Print and shaded views of the part. All mm, measured from the part's lowest x, y and z. A direction names the side the tool comes from. Round coordinates to 2 decimals unless told otherwise and drop trailing zeros. Write each loop counter-clockwise with the first axis right and the second up, starting at its lowest first coordinate (ties: lowest second). Pieces come first, ordered by that corner, then holes. Notation, with made-up numbers: (88, 10.25) - (139, 10.25) arc R31 cw to (139, 41.25) - close; hole circle Ø6 at (25.25, 6.5). An arc over 180 degrees is marked (long way). One line per item, written item: value.
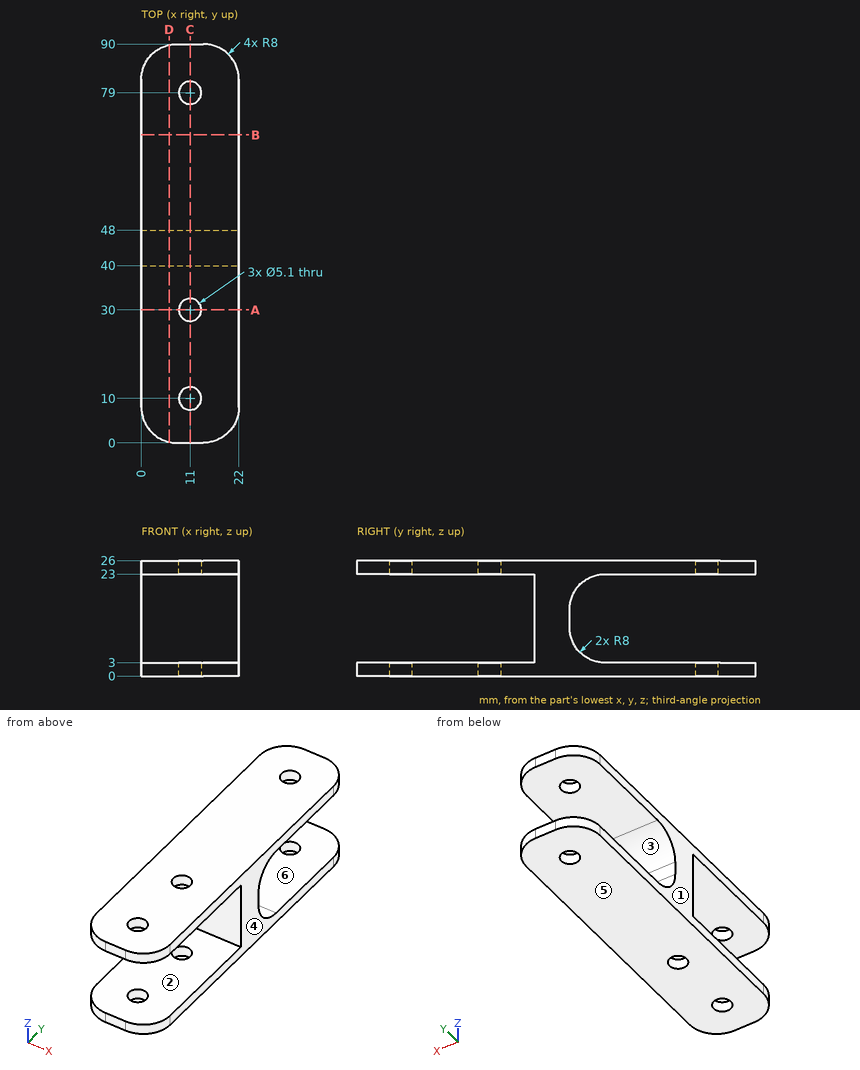
1. Band-saw the part on A-A on y = 30. Write the cut outline in (x, z), plus the area to 3 significant figures.
Report:
outline: (0, 0) - (8.45, 0) - (8.45, 3) - (0, 3) - close; (0, 23) - (8.45, 23) - (8.45, 26) - (0, 26) - close; (13.55, 0) - (22, 0) - (22, 3) - (13.55, 3) - close; (13.55, 23) - (22, 23) - (22, 26) - (13.55, 26) - close
area: 101 mm²
2. Band-saw the part on B-B on y = 69.5. Write the cut outline in (x, z), plus the area to 3 significant figures.
Report:
outline: (0, 0) - (22, 0) - (22, 3) - (0, 3) - close; (0, 23) - (22, 23) - (22, 26) - (0, 26) - close
area: 132 mm²
3. Band-saw the part on D-D on x = 6.25. Write the cut outline in (y, z), plus the area to 3 significant figures.
Report:
outline: (0.19, 0) - (89.81, 0) - (89.81, 3) - (56, 3) arc R8 cw to (48, 11) - (48, 15) arc R8 cw to (56, 23) - (89.81, 23) - (89.81, 26) - (0.19, 26) - (0.19, 23) - (40, 23) - (40, 3) - (0.19, 3) - close
area: 725 mm²
4. Drop flat-ended pins along their axis: pin 1 (11 mm diameter, centred on x = 10, y = 76.5, fed in from -Z); pin 2 (1.2 mm diameter, centred on x = 10, z = 14, fed in from +Y); pin 3 (4 mm diameter, centred on x = 14, z = 8.5, fed in from -Y). Give the stop position or say it passes through.
Report:
pin 1: z = 0
pin 2: y = 48
pin 3: y = 40
5. Mould opens along Z. For the marked faces 4, 5 and 6 say: released by +Z, released by -Z, zero draft, split by the parting line, or undercut.
Report:
face 4: zero draft
face 5: released by -Z
face 6: undercut
6. Band-saw the part on C-C on x = 11. State how many separate pieces and enclosed holes the cut face has, plus the area to 3 significant figures.
Report:
separate pieces: 7
enclosed holes: 0
area: 636 mm²
7. Tool access for the marked faces 1, 2 and 3: list every direction of +Z, -Z, +X, -X, +Y, -Y with a clear straight run to the whole face (end or side of a thin tool).
Report:
face 1: +Z, -Z, -X, +Y, -Y
face 2: +X, -X, -Y
face 3: +X, -X, +Y
8. Wall check: probe 1 along Y at (x, z) = (11, 25.3); probe 2 along Z at (x, y) = (12, 82); probe 3 along Y at (x, z) = (2, 13). Give the ranges that are in metal, low to high. Write a range as [from, to].
Report:
probe 1: [0, 7.45], [12.55, 27.45], [32.55, 76.45], [81.55, 90]
probe 2: [0, 3], [23, 26]
probe 3: [40, 48]
